Read the model definition and answer for the solid it produces. Units are mm, in the model's axes. A direction names the side the tool comes from. Round coordinates to 2 decimals unless told otherwise and drop trailing zeros.
from build123d import *

# Parameters (mm, degrees)
BOSS_EXTRUDE3_OUTLINE_R = 3
BOSS_EXTRUDE3_DEPTH     = 102
CUT_EXTRUDE1_DEPTH      = 102
CUT_EXTRUDE2_DEPTH      = 102
SKETCH4_W               = 0.4
SKETCH4_H               = 1.8
SKETCH4_W_2             = 1.8
SKETCH4_H_2             = 0.4
BOSS_EXTRUDE4_DEPTH     = 102
SKETCH5_W               = 75
SKETCH5_H               = 43.392810524
CUT_EXTRUDE6_DEPTH      = 10
SKETCH7_R               = 3.05
CUT_EXTRUDE9_DEPTH      = 147.084376475
CUT_EXTRUDE8_START      = -102
CUT_EXTRUDE8_DEPTH      = 102
FILLET1_R               = 4


# Read off the part's stored shape, not the designer's step: Boss-Extrude3
with BuildPart() as part:
    # Boss-Extrude3 outline → Boss-Extrude3 (new body)
    with BuildSketch(Plane.XY):
        with BuildLine():
            add(Edge.make_bspline(
                [(24.392810524, -72.348554199), (27.040667073, -69.541086329), (29.089162938, -67.428574969), (30.241441862, -64.355831171), (31.073643307, -60.963009895), (30.561519341, -59.042545022), (29.217193929, -56.673971678), (27.488775543, -54.241382838), (25.105954954, -53), (17.37432721, -53), (-19, -52.782560411)],
                knots=[0, 0, 0, 0, 0, 0, 0, 0, 0, 0, 0, 1, 1, 1, 1, 1, 1, 1, 1, 1, 1, 1], degree=10))
            ThreePointArc((24.392810524, -72.348554199), (55.939709188, -51.962211615), (73.948106805, -19))
            Line((73.948106805, -19), (52.782560411, -19))
            add(Edge.make_bspline(
                [(72.348554199, 24.392810524), (69.541086329, 27.040667073), (67.428574969, 29.089162938), (64.355831171, 30.241441862), (60.963009895, 31.073643307), (59.042545022, 30.561519341), (56.673971678, 29.217193929), (54.241382838, 27.488775543), (53, 25.105954954), (53, 17.37432721), (52.782560411, -19)],
                knots=[0, 0, 0, 0, 0, 0, 0, 0, 0, 0, 0, 1, 1, 1, 1, 1, 1, 1, 1, 1, 1, 1], degree=10))
            ThreePointArc((72.348554199, 24.392810524), (51.962211615, 55.939709188), (19, 73.948106805))
            Line((19, 73.948106805), (19, 53))
            add(Edge.make_bspline(
                [(-24.392810524, 72.348554199), (-27.040667073, 69.541086329), (-29.089162938, 67.428574969), (-30.241441862, 64.355831171), (-31.073643307, 60.963009895), (-30.561519341, 59.042545022), (-29.217193929, 56.673971678), (-27.488775543, 54.241382838), (-25.105954954, 53), (-17.37432721, 53), (19, 53)],
                knots=[0, 0, 0, 0, 0, 0, 0, 0, 0, 0, 0, 1, 1, 1, 1, 1, 1, 1, 1, 1, 1, 1], degree=10))
            ThreePointArc((-24.392810524, 72.348554199), (-55.939709188, 51.962211615), (-73.948106805, 19))
            Line((-73.948106805, 19), (-52.782560411, 19))
            add(Edge.make_bspline(
                [(-72.348554199, -24.392810524), (-69.541086329, -27.040667073), (-67.428574969, -29.089162938), (-64.355831171, -30.241441862), (-60.963009895, -31.073643307), (-59.042545022, -30.561519341), (-56.673971678, -29.217193929), (-54.241382838, -27.488775543), (-53, -25.105954954), (-53, -17.37432721), (-52.782560411, 19)],
                knots=[0, 0, 0, 0, 0, 0, 0, 0, 0, 0, 0, 1, 1, 1, 1, 1, 1, 1, 1, 1, 1, 1], degree=10))
            ThreePointArc((-72.348554199, -24.392810524), (-51.962211615, -55.939709188), (-19, -73.948106805))
            Line((-19, -73.948106805), (-19, -52.782560411))
        make_face()
        with Locations((-30, -58.782560411)):
            Circle(BOSS_EXTRUDE3_OUTLINE_R, mode=Mode.SUBTRACT)
        with Locations((58.782560411, -30)):
            Circle(BOSS_EXTRUDE3_OUTLINE_R, mode=Mode.SUBTRACT)
        with Locations((-58.782560411, 30)):
            Circle(BOSS_EXTRUDE3_OUTLINE_R, mode=Mode.SUBTRACT)
        Polygon((-38.9, -51.6), (-51.6, -51.6), (-51.6, -38.9), (-50, -38.9), (-50, 38.9), (-51.6, 38.9), (-51.6, 51.6), (-38.9, 51.6), (-38.9, 50), (38.9, 50), (38.9, 51.6), (51.6, 51.6), (51.6, 38.9), (50, 38.9), (50, -38.9), (51.6, -38.9), (51.6, -51.6), (38.9, -51.6), (38.9, -50), (-38.9, -50), align=None, mode=Mode.SUBTRACT)
        with Locations((30, 59)):
            Circle(BOSS_EXTRUDE3_OUTLINE_R, mode=Mode.SUBTRACT)
    extrude(amount=BOSS_EXTRUDE3_DEPTH)

    # Sketch2 → Cut-Extrude1 (cut)
    with BuildSketch(Plane.XY.offset(102)):
        Polygon((51.8, -38.7), (50.2, -38.7), (50.2, 38.7), (51.8, 38.7), (51.8, 51.8), (38.7, 51.8), (38.7, 50.2), (-38.7, 50.2), (-38.7, 51.8), (-51.8, 51.8), (-51.8, 38.7), (-50.2, 38.7), (-50.2, -38.7), (-51.8, -38.7), (-51.8, -51.8), (-38.7, -51.8), (-38.7, -50.2), (38.7, -50.2), (38.7, -51.8), (51.8, -51.8), align=None)
        Polygon((51.6, -38.9), (50, -38.9), (50, 38.9), (51.6, 38.9), (51.6, 51.6), (38.9, 51.6), (38.9, 50), (-38.9, 50), (-38.9, 51.6), (-51.6, 51.6), (-51.6, 38.9), (-50, 38.9), (-50, -38.9), (-51.6, -38.9), (-51.6, -51.6), (-38.9, -51.6), (-38.9, -50), (38.9, -50), (38.9, -51.6), (51.6, -51.6), align=None, mode=Mode.SUBTRACT)
    extrude(amount=-CUT_EXTRUDE1_DEPTH, mode=Mode.SUBTRACT)

    # Sketch3 → Cut-Extrude2 (cut)
    with BuildSketch(Plane.XY.offset(102)):
        Polygon((-51.8, -51.8), (-38.7, -51.8), (-38.7, -52), (-52, -52), (-52, -38.7), (-51.8, -38.7), align=None)
        Polygon((38.7, -51.8), (51.8, -51.8), (51.8, -38.7), (52, -38.7), (52, -52), (38.7, -52), align=None)
        Polygon((51.8, 38.7), (51.8, 51.8), (38.7, 51.8), (38.7, 52), (52, 52), (52, 38.7), align=None)
        Polygon((-51.8, 51.8), (-51.8, 38.7), (-52, 38.7), (-52, 52), (-38.7, 52), (-38.7, 51.8), align=None)
    extrude(amount=-CUT_EXTRUDE2_DEPTH, mode=Mode.SUBTRACT)

    # Sketch4 → Boss-Extrude4 (add)
    with BuildSketch(Plane.XY.offset(102)):
        with Locations((-38.9, 51.1)):
            Rectangle(SKETCH4_W, SKETCH4_H)
        with Locations((-51.1, 38.9)):
            Rectangle(SKETCH4_W_2, SKETCH4_H_2)
        with Locations((38.9, 51.1)):
            Rectangle(SKETCH4_W, SKETCH4_H)
        with Locations((51.1, 38.9)):
            Rectangle(SKETCH4_W_2, SKETCH4_H_2)
        with Locations((38.9, -51.1)):
            Rectangle(SKETCH4_W, SKETCH4_H)
        with Locations((51.1, -38.9)):
            Rectangle(SKETCH4_W_2, SKETCH4_H_2)
        with Locations((-51.1, -38.9)):
            Rectangle(SKETCH4_W_2, SKETCH4_H_2)
        with Locations((-38.9, -51.1)):
            Rectangle(SKETCH4_W, SKETCH4_H)
    extrude(amount=-BOSS_EXTRUDE4_DEPTH)

    # Sketch5 → Cut-Extrude6 (cut)
    with BuildSketch(Plane.ZY.offset(-50.2)):
        with Locations((49, 2.696405262)):
            Rectangle(SKETCH5_W, SKETCH5_H)
    extrude(amount=-CUT_EXTRUDE6_DEPTH, mode=Mode.SUBTRACT)

    # Sketch7 → Cut-Extrude9 (cut, through all)
    with BuildSketch(Plane(origin=(0, 0, 0), x_dir=(-1, 0, 0), z_dir=(0, 0, -1))):
        with Locations((30, -58.782560411)):
            Circle(SKETCH7_R)
        with Locations((-58.782560411, -30)):
            Circle(SKETCH7_R)
        with Locations((58.782560411, 30)):
            Circle(SKETCH7_R)
        with Locations((-30, 59)):
            Circle(SKETCH7_R)
    extrude(amount=-CUT_EXTRUDE9_DEPTH, mode=Mode.SUBTRACT)

    # Sketch6 → Cut-Extrude8 (cut)
    with BuildSketch(Plane.XY.offset(102).offset(CUT_EXTRUDE8_START)):
        with BuildLine():
            ThreePointArc((-65.806507446, 38.714675225), (-63.755574673, 39.214145383), (-64.234874045, 41.269885588))
            ThreePointArc((-64.234874045, 41.269885588), (-65.0332415, 40), (-65.806507446, 38.714675225))
        make_face()
        with BuildLine():
            ThreePointArc((-38.714675225, 65.806507446), (-40, 65.0332415), (-41.269885588, 64.234874045))
            ThreePointArc((-41.269885588, 64.234874045), (-39.214145383, 63.755574673), (-38.714675225, 65.806507446))
        make_face()
        with BuildLine():
            ThreePointArc((41.269885588, 64.234874045), (40, 65.0332415), (38.714675225, 65.806507446))
            ThreePointArc((38.714675225, 65.806507446), (39.214145383, 63.755574673), (41.269885588, 64.234874045))
        make_face()
        with BuildLine():
            ThreePointArc((65.806507446, 38.714675225), (65.0332415, 40), (64.234874045, 41.269885588))
            ThreePointArc((64.234874045, 41.269885588), (63.755574673, 39.214145383), (65.806507446, 38.714675225))
        make_face()
        with BuildLine():
            ThreePointArc((65.806507446, -38.714675225), (63.755574673, -39.214145383), (64.234874045, -41.269885588))
            ThreePointArc((64.234874045, -41.269885588), (65.0332415, -40), (65.806507446, -38.714675225))
        make_face()
        with BuildLine():
            ThreePointArc((38.714675225, -65.806507446), (40, -65.0332415), (41.269885588, -64.234874045))
            ThreePointArc((41.269885588, -64.234874045), (39.214145383, -63.755574673), (38.714675225, -65.806507446))
        make_face()
        with BuildLine():
            ThreePointArc((-38.714675225, -65.806507446), (-39.214145383, -63.755574673), (-41.269885588, -64.234874045))
            ThreePointArc((-41.269885588, -64.234874045), (-40, -65.0332415), (-38.714675225, -65.806507446))
        make_face()
        with BuildLine():
            ThreePointArc((-65.806507446, -38.714675225), (-65.0332415, -40), (-64.234874045, -41.269885588))
            ThreePointArc((-64.234874045, -41.269885588), (-63.755574673, -39.214145383), (-65.806507446, -38.714675225))
        make_face()
    extrude(amount=CUT_EXTRUDE8_DEPTH, mode=Mode.SUBTRACT)

    # Fillet1
    fillet1_edges = [part.edges().sort_by_distance(p)[0] for p in [
        (-41.269885588, 64.234874045, 51),
        (-38.714675225, 65.806507446, 51),
        (41.269885588, 64.234874045, 51),
        (38.714675225, 65.806507446, 51),
        (64.234874045, 41.269885588, 51),
        (65.806507446, 38.714675225, 51),
        (64.234874045, -41.269885588, 51),
        (65.806507446, -38.714675225, 51),
        (41.269885588, -64.234874045, 51),
        (38.714675225, -65.806507446, 51),
        (-41.269885588, -64.234874045, 51),
        (-38.714675225, -65.806507446, 51),
        (-64.234874045, -41.269885588, 51),
        (-65.806507446, -38.714675225, 51),
        (-64.234874045, 41.269885588, 51),
        (-65.806507446, 38.714675225, 51),
    ]]
    fillet(fillet1_edges, radius=FILLET1_R)


solid = part.part
Q1. For faces 1 (the face through (-52, 45, 52)), 2 (the face through (51, 2, 11.5)), 3 (the face through (19, 64, 50)), 4 (the face through (30.55, -69.97, 50.29)), determine the directions among +Z, -Z, +X, -X, +Y, -Y from which every point of the face is accessible in a straight line to the end or side of a thin tool.
Outcome:
face 1: +Z, -Z
face 2: +X
face 3: +Z, -Z, +Y
face 4: +Z, -Z, +X, -Y
Q2. A cutting plane is placed at A-A, the plane y = 15.5. Give the number of separate pieces and of enclosed holes in the cut face, plus the area to 3 significant figures.
Outcome:
separate pieces: 3
enclosed holes: 0
area: 352 mm2
Q3. Straight lines are drawn through the part: probe 1 along X at (y, z) = (-61, 93.5); probe 2 along X at (y, z) = (-59.5, 6.5); probe 3 along Y at (x, z) = (-33.5, 18). For each, find the intervals that lie inside material, in ascending order.
Outcome:
probe 1: x = -45.92 to -32.09, -27.91 to -19, 29.87 to 45.92
probe 2: x = -47.84 to -32.96, -27.04 to -19, 29.58 to 47.84
probe 3: y = -68.61 to -50.2, 50.2 to 68.61
Q4. For a pull along Z with two mould halves and no side action, classify faces 5 (the face through (50.2, -27, 52)), 6 (the face through (54, -22, 0)), 7 (the face through (51, 2, 86.5)), 8 (the face through (54, -22, 102)) as released by +Z, released by -Z, zero draft, split by the parting line, or undercut.
Outcome:
face 5: zero draft
face 6: released by -Z
face 7: undercut
face 8: released by +Z
Q5. Flat-ended cylindrical pins translate along their axes: pin 1 (8 mm diameter, centred on y = 23, z = 29, fed in from +X); pin 2 (0.5 mm diameter, centred on y = -51.5, z = 50, fed in from +X); pin 3 (2 mm diameter, centred on y = 51.5, z = 72.5, fed in from +X). Find the tip coordinate at first contact, or state that the pin passes through.
Outcome:
pin 1: stops at x = 72.35
pin 2: stops at x = 56.59
pin 3: stops at x = 57.26
